from build123d import *

# Parameters (mm, degrees)
CONG_1_R = 0.3


with BuildPart() as part:
    # Esquisse1 → Base-Révolution (revolve)
    with BuildSketch(Plane.XY):
        with BuildLine():
            Line((0, 5.25), (1.381966011, 5.25))
            ThreePointArc((1.381966011, 5.25), (2.5, 5.75), (3.618033989, 5.25))
            Line((3.618033989, 5.25), (5, 5.25))
            Line((5, 5.25), (5, 6.5))
            Line((5, 6.5), (0, 6.5))
            Line((0, 6.5), (0, 5.25))
        make_face()
    revolve(axis=Axis((0, 0, 0), (1, 0, 0)))

    # Congé1
    cong_1_edges = [part.edges().sort_by_distance(p)[0] for p in [
        (5, -6.5, 0),
        (0, -6.5, 0),
    ]]
    fillet(cong_1_edges, radius=CONG_1_R)


solid = part.part
Verification items for the finished model (mm, model axes). Coordinates: 2 decimals unless noted, no trailing zeros. Loops run counter-clockwise (first coordinate to the right, second up) from the corner with the lowest first, then second, coordinate; pieces in that order, holes last. Notation, with made-up numbers: M 11,22 L 58,22 A11 ccw 58,34 Z; hole C 76,27 d8. An arc over 180 degrees is marked long. One line per item, written item: value.
1. Material ranges on line 1 along Z through (x, y) = (4.15, 0); line 2 along X through (y, z) = (0, 6.25); line 3 along Z through (x, y) = (2.8, -1.75), recorded low to high. Write a range as from..to.
Answers follow:
line 1: -6.5..-5.25, 5.25..6.5
line 2: 0..5
line 3: -6.26..-5.45, 5.45..6.26
2. Mould release check, pull along Y, two halves, no side actions. Record for faces 1 (the cylindrical face through (2.469, -5.158, -3.955)), 2 (the flat face through (5, 5, 3)), 3 (the cylindrical face through (4.3, 5, 1.6)): pulls with the +Y half, pulls with the -Y half, needs draft (parallel to the pull), parting line crosses it, or undercut.
Answers follow:
face 1: parting line crosses it
face 2: needs draft
face 3: undercut
3. Section check D-D on x = 3.15. Record the cut outline in (y, z), plus the area to 3 significant figures.
Answers follow:
outline: C 0,0 d13; hole C 0,0 d11.2
area: 34.1 mm^2
4. Section check A-A on y = 0. Record the cut outline in (x, z), plus the area to 3 significant figures.
Answers follow:
outline: M 0,-6.2 A0.3 ccw 0.3,-6.5 L 4.7,-6.5 A0.3 ccw 5,-6.2 L 5,-5.25 L 3.62,-5.25 A1.5 cw 1.38,-5.25 L 0,-5.25 Z; M 0,5.25 L 1.38,5.25 A1.5 cw 3.62,5.25 L 5,5.25 L 5,6.2 A0.3 ccw 4.7,6.5 L 0.3,6.5 A0.3 ccw 0,6.2 Z
area: 10.9 mm^2
5. Section check C-C on x = 1.15. Record the cut outline in (y, z), plus the area to 3 significant figures.
Answers follow:
outline: C 0,0 d13; hole C 0,0 d10.5
area: 46.1 mm^2
